Can you work these out from the model? Positions are in its coordinate system, mm. Face numbers are marked on the shaded views. A direction names the side the tool comes from. Give positions to 0.01 mm unless a question says otherwise; leave off trailing zeros. Order: outer loops, then holes, each group sorted by start corner. A loop starts at its lowest first (then second) coordinate and runs counter-clockwise, first axis right, second up. Notation, with made-up numbers: (41, 26.5) - (91, 26.5) arc R35 ccw to (91, 62.5) - close; hole circle Ø10 at (48, 75). An arc over 180 degrees is marked (long way). Use one line per item in the form item = value. Start each with the question number.
1) Please list where these lines run through material, in increasing order: probe 1 along Z at (x, y) = (-56.5, 25.5); probe 2 along Z at (x, y) = (72, 140); probe 3 along X at (y, z) = (-92, 247.5).
2) Suppose I cut it at C-C, the plane x = 102.5. Write out the boundary of the cut face in (y, z), and give its area (3 significant figures).
3) Suppose I cut it at B-B, the plane z = 113.5. Write out the boundary of the cut face in (x, y).
4) Suppose I cut it at D-D, the plane z = 233.5. Write out the boundary of the cut face in (x, y), and give its area (3 significant figures).
5) For pin 1 (3 mm diameter, centred on x = 95.5, y = -53.5, fed in from +Z); pin 2 (4 mm diameter, centred on x = 99.5, y = -48.5, fed in from +Z); pin 3 (1 mm diameter, centred on y = -36.5, z = 106, fed in from -X), each with a flat end and sliding along its axis, tell me the tip position at first contact or that it passes through.
6) Suppose I cut it at A-A, the plane y = 86.5. Write out the boundary of the cut face in (x, z), and give its area (3 significant figures).
7) Which directions (+Z, -Z, +X, -X, +Y, -Y) give clear straight access to the entire face, cutting with the end or side of a thin tool? Please do the marked faces 1 and 2.
```python
from build123d import *

# Parameters (mm, degrees)
F0_W     = 265.33243
F0_H     = 337.1588
F1_DEPTH = 269.24
F3_DEPTH = 346.71
F5_DEPTH = 110.744


with BuildPart() as f1:
    # F0 (on Top) → F1 (new body)
    with BuildSketch(Plane.XY):
        Rectangle(F0_W, F0_H)
    extrude(amount=F1_DEPTH)

    # F2 (on face) → F3 (cut)
    with BuildSketch(Plane(origin=(0, 168.5794, 0), x_dir=(-1, 0, 0), z_dir=(0, 1, 0))):
        Polygon((-132.666215, 91.44), (-56.466215, 269.24), (-132.666215, 269.24), align=None)
        Polygon((56.466215, 0), (132.666215, 0), (132.666215, 177.8), align=None)
    extrude(amount=-F3_DEPTH, mode=Mode.SUBTRACT)

    # F4 (on face) → F5 (cut)
    with BuildSketch(Plane(origin=(0, 168.5794, 0), x_dir=(-1, 0, 0), z_dir=(0, 1, 0))):
        Polygon((132.666215, 177.8), (132.666215, 206.214771), (44.288456, 0), (56.466215, 0), align=None)
    extrude(amount=-F5_DEPTH, mode=Mode.SUBTRACT)


solid = f1.part
```
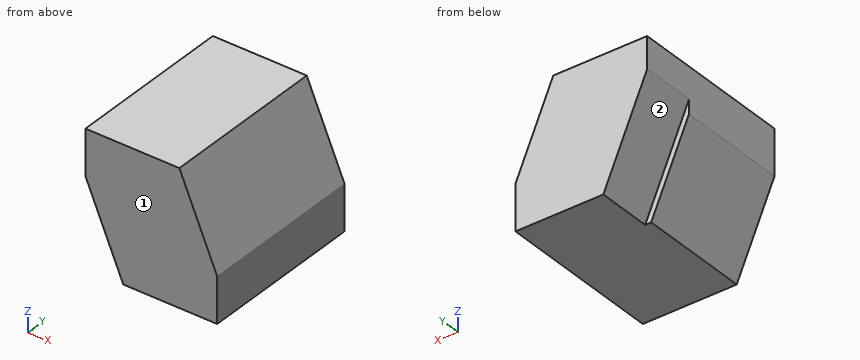
Result sheet:
q1.probe_1 = 0.08 to 269.24
q1.probe_2 = 0 to 232.99
q1.probe_3 = -132.67 to 65.78
q2.outline = (-168.58, 0) - (168.58, 0) - (168.58, 161.83) - (-168.58, 161.83) - close
q2.area = 54,600 mm²
q3.outline = (-105.11, -168.58) - (123.21, -168.58) - (123.21, 168.58) - (-92.93, 168.58) - (-92.93, 57.84) - (-105.11, 57.84) - close
q4.outline = (-132.67, -168.58) - (71.78, -168.58) - (71.78, 168.58) - (-132.67, 168.58) - close
q4.area = 68,900 mm²
q5.pin_1 = 181.66
q5.pin_2 = 173.49
q5.pin_3 = -102.11
q6.outline = (-132.67, 206.21) - (-44.29, 0) - (132.67, 0) - (132.67, 91.44) - (56.47, 269.24) - (-132.67, 269.24) - close
q6.area = 55,600 mm²
q7.face_1 = +Z, -Z, +X, -X, -Y
q7.face_2 = -Z, -X, +Y
